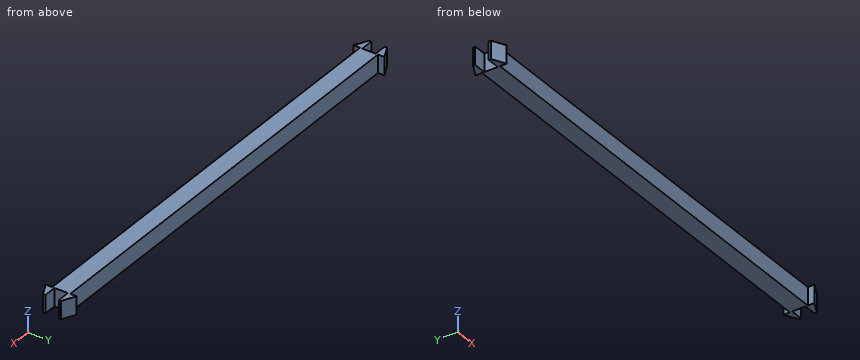
from build123d import *

# Parameters (mm, degrees)
F1_DEPTH = 8.8
F2_DEPTH = 25
F3_DEPTH = 25


with BuildPart() as f1:
    # F0 (on Top) → F1 (new body)
    with BuildSketch(Plane.XY):
        Polygon((107.95, 4.459752), (0, 4.459752), (-107.95, 4.459752), (-107.95, 3.359752), (-107.95, -3.240248), (-107.95, -4.340248), (107.95, -4.340248), (107.95, -3.240248), (107.95, 0), (107.95, 0.059752), (107.95, 3.359752), align=None)
        Polygon((-107.95, 3.359752), (-107.95, 4.459752), (-107.95, 7.634752), (-114.3, 4.459752), (-114.3, 3.359752), align=None)
        Polygon((107.95, 7.634752), (107.95, 4.459752), (107.95, 3.359752), (114.3, 3.359752), (114.3, 4.4), align=None)
        Polygon((-107.95, -3.240248), (-107.95, 3.359752), (-114.3, 3.359752), (-114.3, 0.059752), (-114.3, -3.240248), align=None)
        Polygon((114.3, 3.359752), (107.95, 3.359752), (107.95, 0.059752), (107.95, 0), (107.95, -3.240248), (114.3, -3.240248), (114.3, 0), align=None)
        Polygon((-107.95, -4.340248), (-107.95, -3.240248), (-114.3, -3.240248), (-114.3, -4.340248), (-107.95, -7.515248), align=None)
        Polygon((107.95, -3.240248), (107.95, -4.340248), (107.95, -7.515248), (114.3, -4.4), (114.3, -3.240248), align=None)
    extrude(amount=-F1_DEPTH)

    # F0 (on Top) → F2 (cut)
    with BuildSketch(Plane.XY):
        Polygon((-107.95, -3.240248), (-107.95, 3.359752), (-114.3, 3.359752), (-114.3, 0.059752), (-114.3, -3.240248), align=None)
    extrude(amount=-F2_DEPTH, mode=Mode.SUBTRACT)

    # F0 (on Top) → F3 (cut)
    with BuildSketch(Plane.XY):
        Polygon((114.3, 3.359752), (107.95, 3.359752), (107.95, 0.059752), (107.95, 0), (107.95, -3.240248), (114.3, -3.240248), (114.3, 0), align=None)
    extrude(amount=-F3_DEPTH, mode=Mode.SUBTRACT)


solid = f1.part
Geometry: final body of the model. Coordinates: model frame, mm. Coordinates: 2 decimals unless noted, no trailing zeros. Loops run counter-clockwise (first coordinate to the right, second up) from the corner with the lowest first, then second, coordinate; pieces in that order, holes last. Notation, with made-up numbers: (-28, -21) - (25, -21) arc R15 cw to (25, 0) - close; hole circle Ø3 at (48.25, 30.25). An arc over 180 degrees is marked (long way). Put each result on its own line as item: value. Start each with the question number.
Q1. Cut plane B-B, the plane x = 15. Return loops of the section in (y, z), and give its area (3 significant figures).
Q2. Pin query (flat end, axial travel): pin 1 Ø3 at (x, z) = (111.5, -2.5) entering from -Y; pin 2 Ø3 at (x, z) = (112.5, -6) entering from +Y; pin 3 Ø2.5 at (y, z) = (6.5, -3) entering from -X. Return the tip coordinate at first contact, or that it passes through.
Q3. Cut plane A-A, the plane z = -5.5. Return loops of the section in (x, y), and give its area (3 significant figures).
Q4. Cut plane C-C, the plane y = -0.25. Return loops of the section in (x, z), and give its area (3 significant figures).
Q5. Line query: line 1 (Y direction, x = 68.5, z = -4); line 2 (X direction, y = 4.5, z = -3.25); line 3 (X direction, y = -5.5, z = -4.5). Output: solid intervals per line, ascending.
Filled sheet:
1. outline: (-4.34, -8.8) - (4.46, -8.8) - (4.46, 0) - (-4.34, 0) - close
1. area: 77.4 mm²
2. pin 1: y = -6.51
2. pin 2: y = 6.08
2. pin 3: x = -112.72
3. outline: (-114.3, -4.34) - (-107.95, -7.52) - (-107.95, -4.34) - (107.95, -4.34) - (107.95, -7.52) - (114.3, -4.4) - (114.3, -3.24) - (107.95, -3.24) - (107.95, 3.36) - (114.3, 3.36) - (114.3, 4.4) - (107.95, 7.63) - (107.95, 4.46) - (-107.95, 4.46) - (-107.95, 7.63) - (-114.3, 4.46) - (-114.3, 3.36) - (-107.95, 3.36) - (-107.95, -3.24) - (-114.3, -3.24) - close
3. area: 1,970 mm²
4. outline: (-107.95, -8.8) - (107.95, -8.8) - (107.95, 0) - (-107.95, 0) - close
4. area: 1,900 mm²
5. line 1: -4.34 to 4.46
5. line 2: -114.22 to -107.95, 107.95 to 114.1
5. line 3: -111.98 to -107.95, 107.95 to 112.06
